The model under review builds one solid part; all positions refer to its coordinate system, in mm. Face numbers are marked on the shaded views. A direction names the side the tool comes from. Give positions to 0.01 mm unless a question says otherwise; leave off trailing zeros. Write each loop counter-clockwise with the first axis right and the second up, starting at its lowest first coordinate (ties: lowest second). Pieces come first, ordered by that corner, then holes. Notation, with made-up numbers: (64.5, 82) -> (103.5, 82) arc R5 cw to (103.5, 87) -> close; hole circle Ø5 at (-35, 6). An arc over 180 degrees is marked (long way). Use CSV: the item, a comma, the result in double quotes.
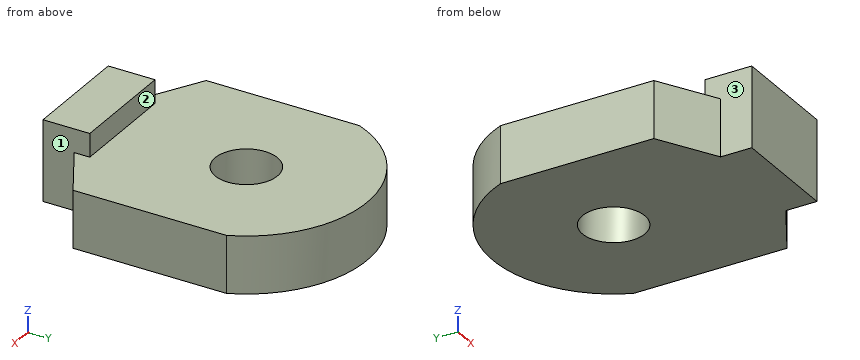
```python
from build123d import *

# Parameters (mm, degrees)
ESQUISSE1_R        = 4
BOSS_EXTRU_1_DEPTH = 7.34
ESQUISSE2_W        = 14
ESQUISSE2_H        = 6
BOSS_EXTRU_2_DEPTH = 3


with BuildPart() as part:
    # Esquisse1 → Boss.-Extru.1 (new body)
    with BuildSketch(Plane.XY):
        with BuildLine():
            Line((-14.29, -13.691116538), (-14.29, 5.977959518))
            ThreePointArc((-14.29, 5.977959518), (0, 15.49), (14.29, 5.977959518))
            Line((14.29, 5.977959518), (14.29, -13.691116538))
            Line((14.29, -13.691116538), (7, -17.9))
            Line((7, -17.9), (7, -21.9))
            Line((7, -21.9), (-7, -21.9))
            Line((-7, -21.9), (-7, -17.9))
            Line((-7, -17.9), (-14.29, -13.691116538))
        make_face()
        Circle(ESQUISSE1_R, mode=Mode.SUBTRACT)
    extrude(amount=BOSS_EXTRU_1_DEPTH)

    # Esquisse2 → Boss.-Extru.2 (add)
    with BuildSketch(Plane.XY.offset(7.34)):
        with Locations((0, -18.9)):
            Rectangle(ESQUISSE2_W, ESQUISSE2_H)
    extrude(amount=BOSS_EXTRU_2_DEPTH)


solid = part.part
```
Q1. Consider section C-C (z = 5.75). Write out the cut boundary in (x, y), then the cut area to 3 significant figures.
Derived:
outline,"(-14.29, -13.69) -> (-7, -17.9) -> (-7, -21.9) -> (7, -21.9) -> (7, -17.9) -> (14.29, -13.69) -> (14.29, 5.98) arc R15.49 ccw to (-14.29, 5.98) -> close; hole circle Ø8 at (0, 0)"
area,"854 mm2"
Q2. Consider section D-D (x = 5). Write out the cut boundary in (y, z), then the cut area to 3 significant figures.
Derived:
outline,"(-21.9, 0) -> (14.66, 0) -> (14.66, 7.34) -> (-15.9, 7.34) -> (-15.9, 10.34) -> (-21.9, 10.34) -> close"
area,"286 mm2"
Q3. Machinability: for the marked faces 1, 2 and 3, which of the approach directions +Z, -Z, +X, -X, +Y, -Y give a long, thin tool a straight path to every point of the face, cutting with its end or side? Answer none if there is none.
Derived:
face 1,"+Z, +X, -Y"
face 2,"+Z, +X, -X, +Y"
face 3,"+Z, -X, -Y"
Q4. Consider section A-A (x = 0). Write out the cut boundary in (y, z), then the cut area to 3 significant figures.
Derived:
outline,"(-21.9, 0) -> (-4, 0) -> (-4, 7.34) -> (-15.9, 7.34) -> (-15.9, 10.34) -> (-21.9, 10.34) -> close; (4, 0) -> (15.49, 0) -> (15.49, 7.34) -> (4, 7.34) -> close"
area,"234 mm2"
Q5. Insertion check: pin 1 (1 mm diameter, centred on x = 11, y = -15.5, fed in from +Z); pin 2 (3 mm diameter, centred on y = -19, z = 5.5, fed in from +X); pin 3 (7 mm diameter, centred on x = 0, y = 0, fed in from -Z); pin 4 (5 mm diameter, centred on y = -20.5, z = 4, fed in from -X). Each pin has a flat end and moves straight along its axis. Give the tip position at first contact, or say it passes through.
Derived:
pin 1,"stops at z = 7.34"
pin 2,"stops at x = 7.69"
pin 3,"passes through"
pin 4,"stops at x = -7"
Q6. To check wall thickness, follow probe 1 along Y at (x, z) = (0, 3.25); probe 2 along Z at (x, y) = (8, -1); probe 3 along X at (y, z) = (-2, 7.25). State the ranges of each line that lie inside material, in increasing order.
Derived:
probe 1,"y = -21.9 to -4, 4 to 15.49"
probe 2,"z = 0 to 7.34"
probe 3,"x = -14.29 to -3.46, 3.46 to 14.29"
Q7. Consider section B-B (y = 0). Write out the cut boundary in (x, z), then the cut area to 3 significant figures.
Derived:
outline,"(-14.29, 0) -> (-4, 0) -> (-4, 7.34) -> (-14.29, 7.34) -> close; (4, 0) -> (14.29, 0) -> (14.29, 7.34) -> (4, 7.34) -> close"
area,"151 mm2"
